Geometry check sheet. Reference: the model listing, model coordinates, mm. A direction names the side the tool comes from. Round coordinates to 2 decimals unless told otherwise and drop trailing zeros. Write each loop counter-clockwise with the first axis right and the second up, starting at its lowest first coordinate (ties: lowest second). Pieces come first, ordered by that corner, then holes. Notation, with made-up numbers: (-17.5, 77) -> (33.5, 77) arc R14 ccw to (33.5, 99) -> close; hole circle Ø11 at (67.5, 41.25). An arc over 180 degrees is marked (long way). Put each result on its own line as item: value. Start each with the question number.
from build123d import *

# Parameters (mm, degrees)
SKETCH_1_R               = 26.5
SKETCH_1_R_2             = 22.5
EXTRUDE_1_DEPTH          = 21
CUT_EXTRUDE_1_DEPTH      = 16
PATTERN_CIRCULAR_1_COUNT = 6
FILLET_1_R               = 1


with BuildPart() as part:
    # 草图1 → 凸台-拉伸1 (new body)
    with BuildSketch(Plane(origin=(0, 0, 0), x_dir=(1, 0, 0), z_dir=(0, 1, 0))):
        with Locations(Location((0, 0, 0), (0, 0, 90))):
            Circle(SKETCH_1_R)
        with Locations(Location((0, 0, 0), (0, 0, 90))):
            Circle(SKETCH_1_R_2, mode=Mode.SUBTRACT)
    extrude(amount=EXTRUDE_1_DEPTH)

    # 草图2 → 切除-拉伸1 (cut)
    with BuildSketch(Plane.XZ):
        with BuildLine():
            ThreePointArc((-1, 22.477766793), (-0.500123564, 22.494441012), (0, 22.5))
            Line((0, 22.5), (0, 24.477766793))
            Line((0, 24.477766793), (-1, 24.477766793))
            Line((-1, 24.477766793), (-1, 22.477766793))
        make_face()
        with BuildLine():
            Line((0, 24.477766793), (0, 22.5))
            ThreePointArc((0, 22.5), (0.500123564, 22.494441012), (1, 22.477766793))
            Line((1, 22.477766793), (1, 24.477766793))
            Line((1, 24.477766793), (0, 24.477766793))
        make_face()
    cut_extrude_1 = extrude(amount=-CUT_EXTRUDE_1_DEPTH, mode=Mode.SUBTRACT)

    # 阵列(圆周)1: 切除-拉伸1 ×6 about axis
    pattern_circular_1_axis = Axis((0, 0, 0), (0, 1, 0))
    for i in range(1, PATTERN_CIRCULAR_1_COUNT):
        add(cut_extrude_1.rotate(pattern_circular_1_axis, i * 360 / PATTERN_CIRCULAR_1_COUNT), mode=Mode.SUBTRACT)

    # 圆角1
    fillet_1_edges = [part.edges().sort_by_distance(p)[0] for p in [
        (0, 0, 26.5),
        (0, 21, 26.5),
    ]]
    fillet(fillet_1_edges, radius=FILLET_1_R)


solid = part.part
(1) Sectioned sample at C-C (y = 3.25). Record the cut outline in (x, z).
(2) Go/stop test with flat-tipped pins: pin 1 Ø5 at (y, z) = (16.5, -4) entering from +X; pin 2 Ø2 at (y, z) = (6.5, -23) entering from -X; pin 3 Ø0.6 at (y, z) = (9.5, -23) entering from +X. Record where each tip stops, or that it passes through.
(3) Sectioned sample at B-B (z = 0). Record the cut outline in (x, y), and give its area (3 significant figures).
(4) Material ranges on L1, parallel to X at y = 4.25, z = 0; L2, parallel to X at y = 4, z = 20.5; L3, parallel to Z at x = 7, y = 14.25, recorded low to high. Write a range as from..to.
(5) Set-up check for faces 1 (the cylindrical face through (-26.274, 10.367, 3.45)), 2 (the flat face through (20, 16, -12)): record each of +Z, -Z, +X, -X, +Y, -Y from which the full face is reachable in a straight line by a thin tool's end or side.
(6) Sectioned sample at D-D (y = 18.25). Record the cut outline in (x, z), and give its area (3 significant figures).
(7) Sectioned sample at A-A (x = 0). Record the cut outline in (y, z), and give its area (3 significant figures).
Found:
1. outline: circle Ø53 at (0, 0); hole (-21.7, -11.37) -> (-20.7, -13.1) -> (-18.97, -12.1) arc R22.5 ccw to (-1, -22.48) -> (-1, -24.48) -> (1, -24.48) -> (1, -22.48) arc R22.5 ccw to (18.97, -12.1) -> (20.7, -13.1) -> (21.7, -11.37) -> (19.97, -10.37) arc R22.5 ccw to (19.97, 10.37) -> (21.7, 11.37) -> (20.7, 13.1) -> (18.97, 12.1) arc R22.5 ccw to (1, 22.48) -> (1, 24.48) -> (-1, 24.48) -> (-1, 22.48) arc R22.5 ccw to (-18.97, 12.1) -> (-20.7, 13.1) -> (-21.7, 11.37) -> (-19.97, 10.37) arc R22.5 ccw to (-19.97, -10.37) -> close
2. pin 1: x = 26.46
2. pin 2: x = -14.77
2. pin 3: x = 13.67
3. outline: (-26.5, 1) arc R1 ccw to (-25.5, 0) -> (-22.5, 0) -> (-22.5, 21) -> (-25.5, 21) arc R1 ccw to (-26.5, 20) -> close; (22.5, 0) -> (25.5, 0) arc R1 ccw to (26.5, 1) -> (26.5, 20) arc R1 ccw to (25.5, 21) -> (22.5, 21) -> close
3. area: 167 mm2
4. L1: -26.5..-22.5, 22.5..26.5
4. L2: -16.79..-9.27, 9.27..16.79
4. L3: -25.56..-21.38, 21.38..25.56
5. face 1: +Y, -Y
5. face 2: -Y
6. outline: circle Ø53 at (0, 0); hole circle Ø45 at (0, 0)
6. area: 616 mm2
7. outline: (0, -25.5) arc R1 ccw to (1, -26.5) -> (20, -26.5) arc R1 ccw to (21, -25.5) -> (21, -22.5) -> (16, -22.5) -> (16, -24.48) -> (0, -24.48) -> close; (0, 24.48) -> (16, 24.48) -> (16, 22.5) -> (21, 22.5) -> (21, 25.5) arc R1 ccw to (20, 26.5) -> (1, 26.5) arc R1 ccw to (0, 25.5) -> close
7. area: 104 mm2
